Answer from the drawing. Dimensions are ordinates in mm from the lowest x, y and z of the part. Give positions to 0.01 mm unless a question says otherwise; leave off trailing zeros. Loops run counter-clockwise (first coordinate to the right, second up) from the corner with the lowest first, then second, coordinate; pieces in that order, holes last. Notation, with made-up numbers: (77.25, -24) - (89.25, -24) arc R28 cw to (89.25, 1) - close; hole circle Ø9 at (-26.5, 21). An arc over 180 degrees is marked (long way). One line per question, with ' | ' between items. Start each with the question number.
1. Find the intervals of material crossed by line 1 (X direction, y = 44, z = 18.5); line 2 (X direction, y = 29, z = 18); line 3 (Z direction, x = 152.5, y = 28), in increasing order.
2. Section C-C (x = 69.5) is taken. Determine the outline of the cut face in (y, z).
3. Each of these flat-tipped pins is pushed along its axis until it touches: pin 1 (23 mm diameter, centred on y = 35.5, z = 15.5, fed in from -X); pin 2 (10 mm diameter, centred on x = 217.5, y = 18.5, fed in from +Z); pin 3 (3 mm diameter, centred on x = 226.5, y = 20.5, fed in from +Z); pin 4 (4 mm diameter, centred on x = 98.5, z = 24, fed in from +Y). Where does it stop, or does it pass through?
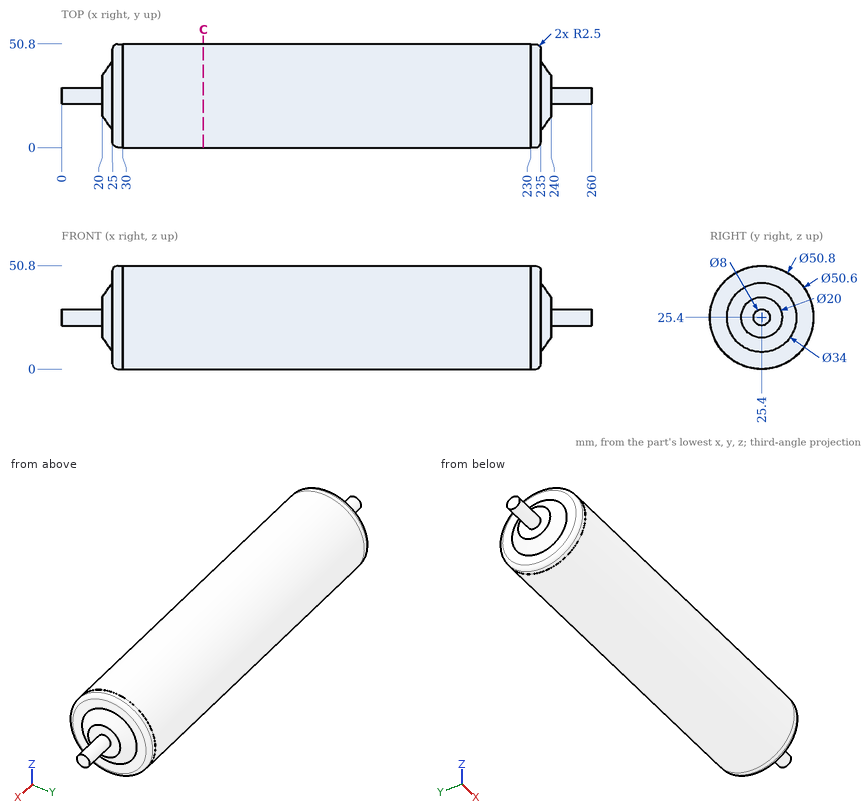
Conclusion:
1) line 1: 25 to 235 | line 2: 20 to 240 | line 3: 0.13 to 50.67
2) outline: circle Ø50.8 at (25.4, 25.4)
3) pin 1: x = 0 | pin 2: z = 50.73 | pin 3: z = 50.57 | pin 4: y = 50.8
